Answer from the drawing. Dimensions are ordinates in mm from the lowest x, y and z of the part. A direction names the side the tool comes from. Coordinates: 2 decimals unless noted, no trailing zeros. Write each loop counter-clockwise with the first axis right and the second up, starting at its lowest first coordinate (ties: lowest second). Pieces come first, ordered by that corner, then holes.
(1) Given P1, Ø0.8, axis at x = 35.5, z = 3, coming from the -Y side; P2, Ø1, axis at y = 12.5, z = 2, coming from the -X side; P3, Ø1, axis at x = 29, z = 5, coming from the +Y side (1 decimal), each flat-ended and moving along its own axis, determine where each tip first touches the part or whether it passes through.
(2) Which of the six approach directions +Z, -Z, +X, -X, +Y, -Y give full straight-line access (tool end or side, diameter ignored) to the marked faces 1 and 2?
(3) The part is cut by section B-B on y = 7. Determine the outline of the cut face in (x, z).
(4) Straight lines are drawn through the part: line 1 (Y direction, x = 33, z = 3) (1 decimal); line 2 (X direction, y = 14, z = 2.25); line 3 (X direction, y = 5.75, z = 2.5). For each, find the intervals that lie inside material, in ascending order.
(5) For a pull along X with two mould halves and no side action, classify the marked faces 3, 4 and 5 as +X half, -X half, draft (parallel to the pull), parting line (faces both ways), or undercut.
(6) The part is cut by section A-A on y = 4.25. Give the number of separate pieces and of enclosed holes in the cut face.
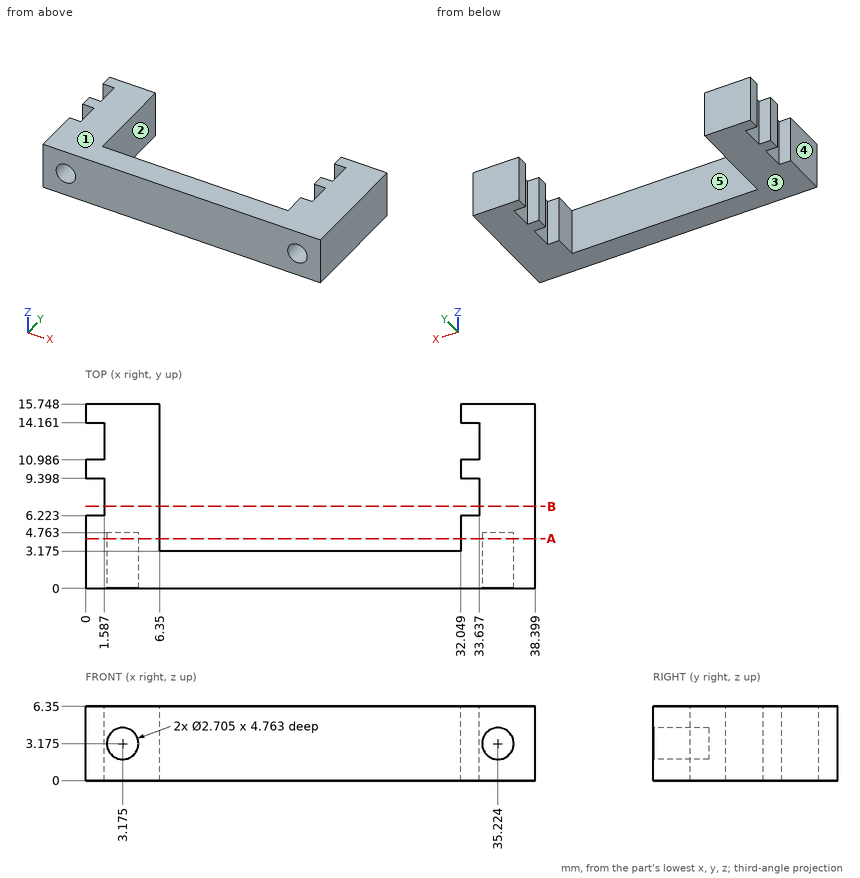
Model answer:
1. P1: stops at y = 4.76
1. P2: stops at x = 1.59
1. P3: stops at y = 3.2
2. face 1: +Z, +X, -X, +Y, -Y
2. face 2: +Z, -Z, +Y
3. outline: (1.59, 0) - (6.35, 0) - (6.35, 6.35) - (1.59, 6.35) - close; (33.64, 0) - (38.4, 0) - (38.4, 6.35) - (33.64, 6.35) - close
4. line 1: y = 0 to 6.2, 9.4 to 11, 14.2 to 15.7
4. line 2: x = 1.59 to 6.35, 33.64 to 38.4
4. line 3: x = 0 to 6.35, 32.05 to 38.4
5. face 3: draft
5. face 4: -X half
5. face 5: undercut
6. separate pieces: 2
6. enclosed holes: 2
